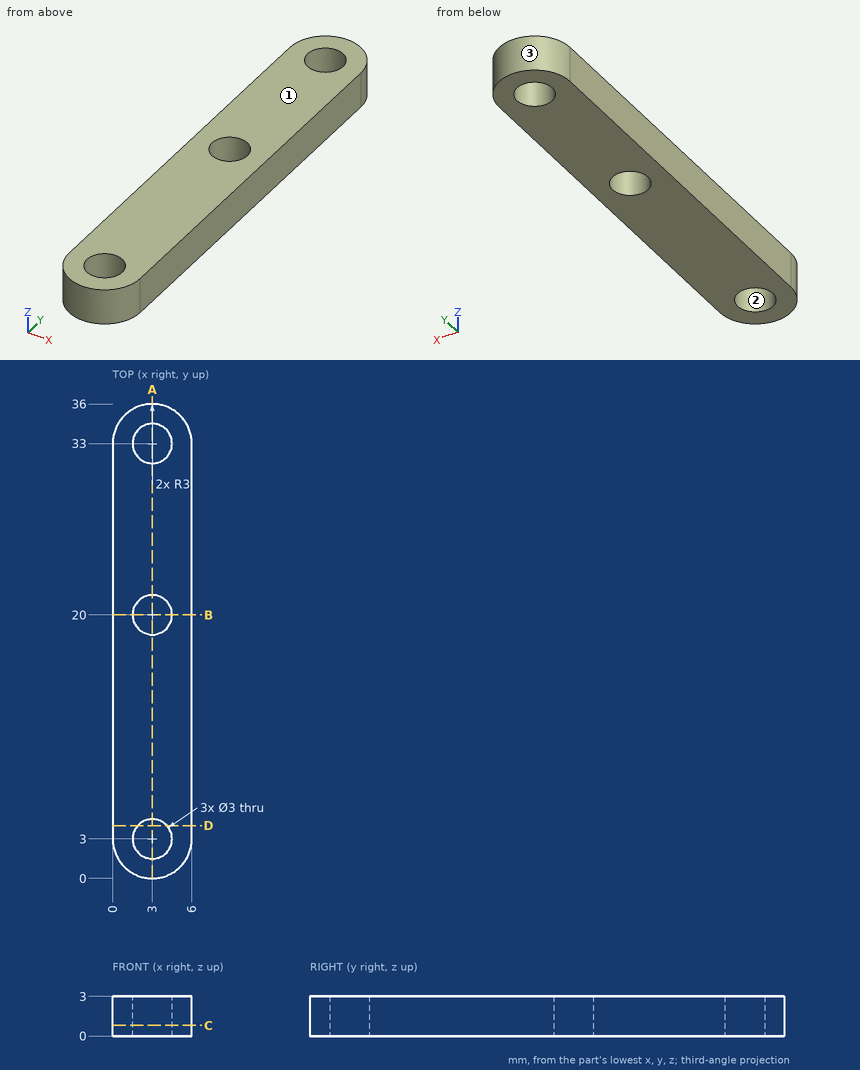
Drawing for the job (mm, zero at the part's lowest x, y, z). Round coordinates to 2 decimals unless told otherwise and drop trailing zeros. Order: outer loops, then holes, each group sorted by start corner. A loop starts at its lowest first (then second) coordinate and runs counter-clockwise, first axis right, second up. Notation, with made-up numbers: (-23, 24.25) -> (29, 24.25) arc R17 cw to (29, 52.25) -> close; hole circle Ø7 at (11, 74). An arc over 180 degrees is marked (long way). Write item = value, one per line. Start each with the question number.
(1) Cut at A-A, the plane x = 3. List the corners of the cut face in (y, z), then the cut area to 3 significant figures.
(2) Pin check, flat tip, straight feed: P1, Ø1, axis at x = 3.5, y = 8.5, coming from the -Z side. Stop position of the tip, or through.
(3) Cut at B-B, the plane y = 20. List the corners of the cut face in (x, z).
(4) Cut at C-C, the plane z = 0.8. List the corners of the cut face in (x, y), then the cut area to 3 significant figures.
(5) Probe line 1 (Y direction, x = 3, z = 1.35); line 2 (Y direction, x = 4, z = 1.85); line 3 (X direction, y = 3, z = 1.1). List the from-to ranges inside material, lowest first. Write a range as [from, to].
(6) Cut at D-D, the plane y = 4. List the corners of the cut face in (x, z).
(7) Pull direction Y, two halves, no side cores. Call the marked faces 1, 2 and 3: released by +Y, released by -Y, zero draft, split by the parting line, or undercut.
Model answer:
q1.outline = (0, 0) -> (1.5, 0) -> (1.5, 3) -> (0, 3) -> close; (4.5, 0) -> (18.5, 0) -> (18.5, 3) -> (4.5, 3) -> close; (21.5, 0) -> (31.5, 0) -> (31.5, 3) -> (21.5, 3) -> close; (34.5, 0) -> (36, 0) -> (36, 3) -> (34.5, 3) -> close
q1.area = 81.0 mm2
q2.P1 = 0
q3.outline = (0, 0) -> (1.5, 0) -> (1.5, 3) -> (0, 3) -> close; (4.5, 0) -> (6, 0) -> (6, 3) -> (4.5, 3) -> close
q4.outline = (0, 3) arc R3 ccw to (6, 3) -> (6, 33) arc R3 ccw to (0, 33) -> close; hole circle Ø3 at (3, 3); hole circle Ø3 at (3, 20); hole circle Ø3 at (3, 33)
q4.area = 187 mm2
q5.line_1 = [0, 1.5], [4.5, 18.5], [21.5, 31.5], [34.5, 36]
q5.line_2 = [0.17, 1.88], [4.12, 18.88], [21.12, 31.88], [34.12, 35.83]
q5.line_3 = [0, 1.5], [4.5, 6]
q6.outline = (0, 0) -> (1.88, 0) -> (1.88, 3) -> (0, 3) -> close; (4.12, 0) -> (6, 0) -> (6, 3) -> (4.12, 3) -> close
q7.face_1 = zero draft
q7.face_2 = undercut
q7.face_3 = released by +Y
